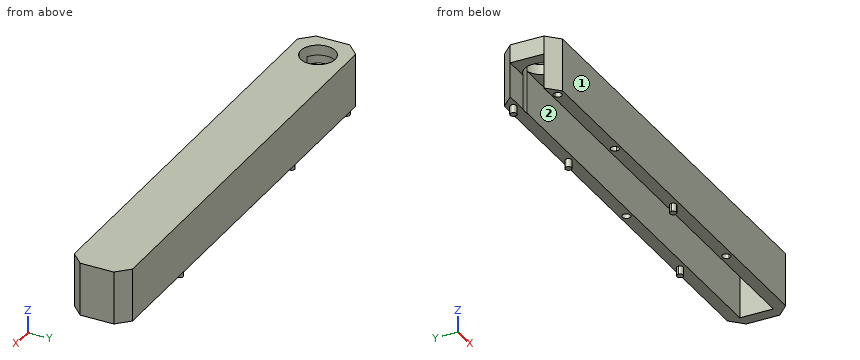
from build123d import *

# Parameters (mm, degrees)
EXTRUDE_5_DEPTH     = 2.5
EXTRUDE_6_DEPTH     = 10.5
SKETCH_6_R          = 1
CUT_EXTRUDE_2_DEPTH = 2
EXTRUDE_7_DEPTH     = 2
SKETCH_8_R          = 0.8
EXTRUDE_8_DEPTH     = 2
CUT_EXTRUDE_3_DEPTH = 2
CUT_EXTRUDE_6_DEPTH = 5
EXTRUDE_9_DEPTH     = 11
EXTRUDE_10_DEPTH    = 11
EXTRUDE_11_DEPTH    = 2
CUT_EXTRUDE_7_DEPTH = 2
SKETCH_19_R         = 0.8
EXTRUDE_13_DEPTH    = 2
SKETCH_20_W         = 8.5
SKETCH_20_H         = 8.2
CUT_EXTRUDE_8_DEPTH = 10


with BuildPart() as part:
    # Sketch 4 → Extrude 5 (new body)
    with BuildSketch(Plane.XY):
        Polygon((52.944203822, -8.2), (52.944203822, 0), (49.944203822, 3), (-54.055796178, 3), (-57.055796178, 0), (-57.055796178, -8.2), (-54.055796178, -11.2), (49.944203822, -11.2), align=None)
        with BuildLine():
            ThreePointArc((-49.14475282, -8.2), (-54.255796178, -4.1), (-49.14475282, 0))
            Line((-49.14475282, 0), (49.944203822, 0))
            Line((49.944203822, 0), (49.944203822, -8.2))
            Line((49.944203822, -8.2), (-49.14475282, -8.2))
        make_face(mode=Mode.SUBTRACT)
        with BuildLine():
            Line((49.944203822, 0), (-49.14475282, 0))
            ThreePointArc((-49.14475282, 0), (-46.77964126, -1.471919151), (-45.855796178, -4.1))
            ThreePointArc((-45.855796178, -4.1), (-46.77964126, -6.728080849), (-49.14475282, -8.2))
            Line((-49.14475282, -8.2), (49.944203822, -8.2))
            Line((49.944203822, -8.2), (49.944203822, 0))
        make_face()
    extrude(amount=EXTRUDE_5_DEPTH)

    # Sketch 4_6 → Extrude 6 (add)
    with BuildSketch(Plane.XY):
        Polygon((52.944203822, -8.2), (52.944203822, 0), (49.944203822, 3), (-54.055796178, 3), (-57.055796178, 0), (-57.055796178, -8.2), (-54.055796178, -11.2), (49.944203822, -11.2), align=None)
        with BuildLine():
            ThreePointArc((-49.14475282, -8.2), (-54.255796178, -4.1), (-49.14475282, 0))
            Line((-49.14475282, 0), (49.944203822, 0))
            Line((49.944203822, 0), (49.944203822, -8.2))
            Line((49.944203822, -8.2), (-49.14475282, -8.2))
        make_face(mode=Mode.SUBTRACT)
    extrude(amount=-EXTRUDE_6_DEPTH)

    # Sketch 6 → Cut-Extrude 2 (cut)
    with BuildSketch(Plane(origin=(0, 0, -10.5), x_dir=(-1, 0, 0), z_dir=(0, 0, -1))):
        with Locations((0.055796178, 1.5)):
            Circle(SKETCH_6_R)
    extrude(amount=-CUT_EXTRUDE_2_DEPTH, mode=Mode.SUBTRACT)

    # Sketch 7 → Extrude 7 (add)
    with BuildSketch(Plane(origin=(0, 0, -10.5), x_dir=(-1, 0, 0), z_dir=(0, 0, -1))):
        with BuildLine():
            ThreePointArc((0.400274499, -9.7), (0.165959924, -9.134314575), (-0.399725501, -8.9))
            Line((-0.399725501, -8.9), (-0.399725501, -10.5))
            ThreePointArc((-0.399725501, -10.5), (0.165959924, -10.265685425), (0.400274499, -9.7))
        make_face()
        with BuildLine():
            Line((-0.399725501, -10.5), (-0.399725501, -8.9))
            ThreePointArc((-0.399725501, -8.9), (-1.199725501, -9.7), (-0.399725501, -10.5))
        make_face()
    extrude(amount=EXTRUDE_7_DEPTH)

    # Sketch 8 → Extrude 8 (add)
    with BuildSketch(Plane(origin=(0, 0, -10.5), x_dir=(-1, 0, 0), z_dir=(0, 0, -1))):
        with BuildLine():
            ThreePointArc((-24.172101911, 1.5), (-24.948107532, 2.299640088), (-25.770662585, 1.547967168))
            Line((-25.770662585, 1.547967168), (-24.173541236, 1.452032832))
            ThreePointArc((-24.173541236, 1.452032832), (-24.172461823, 1.476005621), (-24.172101911, 1.5))
        make_face()
        with BuildLine():
            Line((-24.173541236, 1.452032832), (-25.770662585, 1.547967168))
            ThreePointArc((-25.770662585, 1.547967168), (-25.020069079, 0.701439326), (-24.173541236, 1.452032832))
        make_face()
        with Locations(Location((27.027898089, 1.5, 0), (0, 0, 180))):
            Circle(SKETCH_8_R)
    extrude(amount=EXTRUDE_8_DEPTH)

    # Sketch 9 → Cut-Extrude 3 (cut)
    with BuildSketch(Plane(origin=(0, 0, -10.5), x_dir=(-1, 0, 0), z_dir=(0, 0, -1))):
        with BuildLine():
            ThreePointArc((-24.171964661, -9.7), (-24.172421822, -9.669765703), (-24.173792887, -9.63955905))
            Line((-24.173792887, -9.63955905), (-26.170136436, -9.76044095))
            ThreePointArc((-26.170136436, -9.76044095), (-25.141730364, -10.699542839), (-24.171964661, -9.7))
        make_face()
        with BuildLine():
            Line((-26.170136436, -9.76044095), (-24.173792887, -9.63955905))
            ThreePointArc((-24.173792887, -9.63955905), (-25.232405611, -8.701828225), (-26.170136436, -9.76044095))
        make_face()
        with BuildLine():
            ThreePointArc((27.828035339, -9.7), (26.855549466, -8.700378585), (25.829549393, -9.644992578))
            Line((25.829549393, -9.644992578), (27.826521284, -9.755007422))
            ThreePointArc((27.826521284, -9.755007422), (27.827656754, -9.727514127), (27.828035339, -9.7))
        make_face()
        with BuildLine():
            Line((27.826521284, -9.755007422), (25.829549393, -9.644992578))
            ThreePointArc((25.829549393, -9.644992578), (26.773027917, -10.698485946), (27.826521284, -9.755007422))
        make_face()
    extrude(amount=-CUT_EXTRUDE_3_DEPTH, mode=Mode.SUBTRACT)

    # Sketch 11 → Cut-Extrude 6 (cut)
    with BuildSketch(Plane.ZY.offset(57.055796178)):
        Polygon((0, -8.2), (0, 0), (-10.5, 0), (-10.5, -1.6), (-10.5, -6.6), (-10.5, -8.2), align=None)
    extrude(amount=-CUT_EXTRUDE_6_DEPTH, mode=Mode.SUBTRACT)

    # Sketch 12 → Extrude 9 (add)
    with BuildSketch(Plane(origin=(0, 0, -10.5), x_dir=(-1, 0, 0), z_dir=(0, 0, -1))):
        Polygon((52.055796178, -0.406762937), (57.055796178, 0), (52.055796178, 0), align=None)
    extrude(amount=-EXTRUDE_9_DEPTH)

    # Sketch 13 → Extrude 10 (add)
    with BuildSketch(Plane(origin=(0, 0, -10.5), x_dir=(-1, 0, 0), z_dir=(0, 0, -1))):
        Polygon((52.055796178, -7.793237063), (52.055796178, -8.2), (57.055796178, -8.2), align=None)
    extrude(amount=-EXTRUDE_10_DEPTH)

    # Sketch 15 → Extrude 11 (add)
    with BuildSketch(Plane(origin=(0, 0, 0), x_dir=(-1, 0, 0), z_dir=(0, 0, -1))):
        with BuildLine():
            Line((52.055796178, -0.406762937), (57.055796178, 0))
            Line((57.055796178, 0), (57.055796178, -8.2))
            Line((57.055796178, -8.2), (52.055796178, -7.793237063))
            ThreePointArc((52.055796178, -7.793237063), (54.255796178, -4.1), (52.055796178, -0.406762937))
        make_face()
    extrude(amount=EXTRUDE_11_DEPTH)

    # Sketch 18 → Cut-Extrude 7 (cut)
    with BuildSketch(Plane(origin=(0, 0, -10.5), x_dir=(-1, 0, 0), z_dir=(0, 0, -1))):
        with BuildLine():
            ThreePointArc((54.055796178, -9.496618531), (53.552650389, -8.628784507), (52.549524392, -8.634244553))
            Line((52.549524392, -8.634244553), (53.562067964, -10.35899251))
            ThreePointArc((53.562067964, -10.35899251), (53.923630202, -9.993472742), (54.055796178, -9.496618531))
        make_face()
        with BuildLine():
            Line((53.562067964, -10.35899251), (52.549524392, -8.634244553))
            ThreePointArc((52.549524392, -8.634244553), (52.1934222, -10.002890317), (53.562067964, -10.35899251))
        make_face()
    extrude(amount=-CUT_EXTRUDE_7_DEPTH, mode=Mode.SUBTRACT)

    # Sketch 19 → Extrude 13 (add)
    with BuildSketch(Plane(origin=(0, 0, -10.5), x_dir=(-1, 0, 0), z_dir=(0, 0, -1))):
        with Locations(Location((53.055796178, 1.296618531, 0), (0, 0, 180))):
            Circle(SKETCH_19_R)
    extrude(amount=EXTRUDE_13_DEPTH)

    # Sketch 20 → Cut-Extrude 8 (cut)
    with BuildSketch(Plane.ZY.offset(57.055796178)):
        with Locations((-6.25, -4.1)):
            Rectangle(SKETCH_20_W, SKETCH_20_H)
    extrude(amount=-CUT_EXTRUDE_8_DEPTH, mode=Mode.SUBTRACT)


solid = part.part
Input: part model. Units: mm. Frame: model coordinates. Face numbers are marked on the shaded views. A direction names the side the tool comes from. Coordinates: 2 decimals unless noted, no trailing zeros. Loops run counter-clockwise (first coordinate to the right, second up) from the corner with the lowest first, then second, coordinate; pieces in that order, holes last.
Q1. Cut plane C-C (x = -33). Output: boundary loops of the cut face in (y, z).
Q2. Material intervals for line 1 (Y direction, x = 41, z = -3.5); line 2 (X direction, y = -10, z = -10.25); line 3 (X direction, y = -4.1, z = -1), sorted ascending.
Q3. Cut plane A-A (z = -7.5). Output: boundary loops of the cut face in (x, y).
Q4. Set-up query: the marked faces 1 and 2. Return all of +Z, -Z, +X, -X, +Y, -Y with unobstructed straight access to the full face (end or side cutting, diameter ignored); none if empty.
Q5. Cut plane B-B (y = -2.75). Output: boundary loops of the cut face in (x, z), then the cut area to 3 significant figures.
Q6. Contact query for flat-ended pins moving along their axis: pin 1 (3 mm diameter, centred on x = -55, y = -2.5, fed in from -Z); pin 2 (3 mm diameter, centred on y = -4, z = -7.5, fed in from -X); pin 3 (1.8 mm diameter, centred on x = -55, z = -4.5, fed in from +Y). Output: stop coordinate, or through.
Working result:
1. outline: (-11.2, -10.5) - (-8.2, -10.5) - (-8.2, 0) - (0, 0) - (0, -10.5) - (3, -10.5) - (3, 2.5) - (-11.2, 2.5) - close
2. line 1: y = -11.2 to -8.2, 0 to 3
2. line 2: x = -55.26 to -53.92, -52.19 to -27.78, -25.87 to 24.22, 26.13 to 51.14
2. line 3: x = -57.06 to -54.26, 49.94 to 52.94
3. outline: (-57.06, -8.2) - (-54.06, -11.2) - (49.94, -11.2) - (52.94, -8.2) - (52.94, 0) - (49.94, 3) - (-54.06, 3) - (-57.06, 0) - (-50.97, 0) arc R4.2 cw to (-49.14, 0) - (49.94, 0) - (49.94, -8.2) - (-49.14, -8.2) arc R4.2 cw to (-50.97, -8.2) - close
4. face 1: +Z, -Z, +X, -X, -Y
4. face 2: -Z
5. outline: (-57.06, -2) - (-54.03, -2) - (-54.03, 2.5) - (-57.06, 2.5) - close; (-46.08, 0) - (49.94, 0) - (49.94, -10.5) - (52.94, -10.5) - (52.94, 2.5) - (-46.08, 2.5) - close
5. area: 293 mm2
6. pin 1: stops at z = -2
6. pin 2: stops at x = 49.94
6. pin 3: stops at y = 2.96
